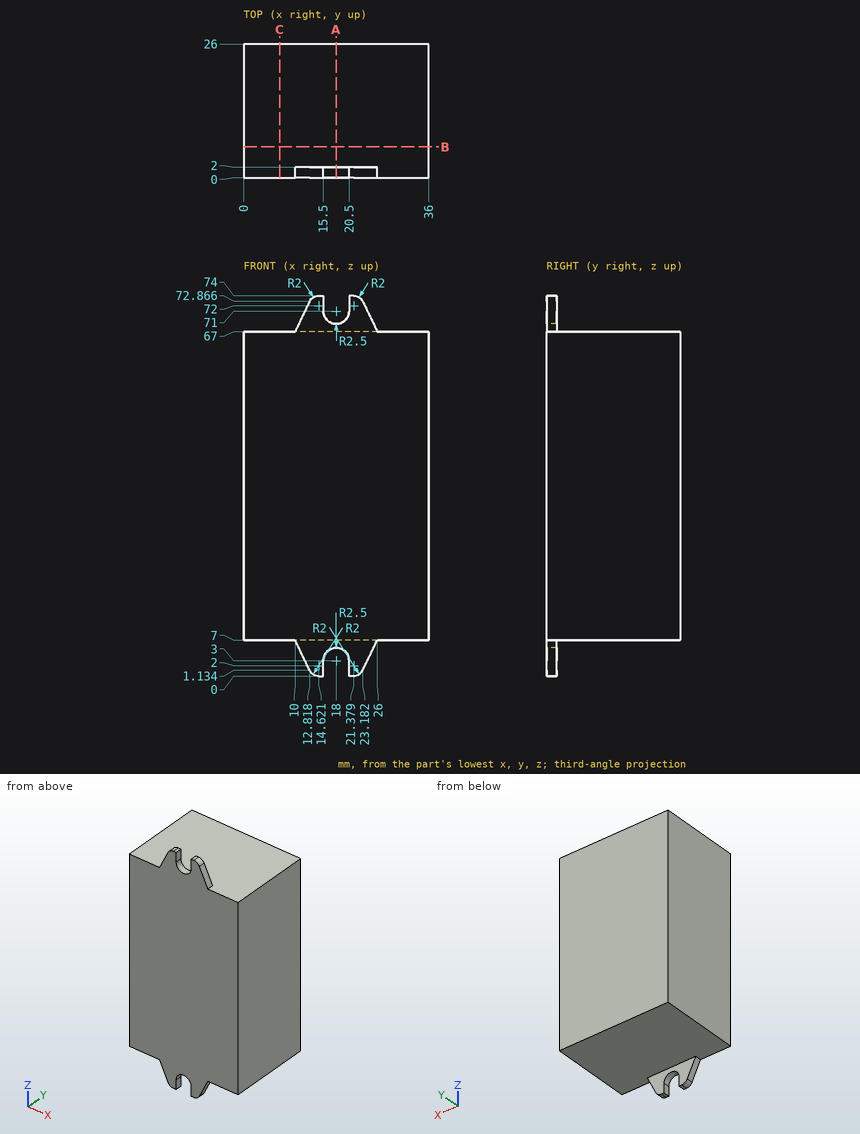
Source: three-view drawing plus pictorial views. Frame: mm from the lowest corner of the part. Round coordinates to 2 decimals unless told otherwise and drop trailing zeros. Order: outer loops, then holes, each group sorted by start corner. A loop starts at its lowest first (then second) coordinate and runs counter-clockwise, first axis right, second up. Notation, with made-up numbers: (47, -0.75) - (85, -0.75) arc R32 cw to (85, 25.25) - close; hole circle Ø11 at (79.25, 9.5). An arc over 180 degrees is marked (long way). Use a Markdown table: item, result.
1. Section C-C on x = 7. Return the cut outline in (y, z).
Evaluation:
| item | result |
|---|---|
| outline | (0, 7) - (26, 7) - (26, 67) - (0, 67) - close |
2. Section B-B on y = 6. Return the cut outline in (x, z), then the cut area to 3 significant figures.
Evaluation:
| item | result |
|---|---|
| outline | (0, 7) - (36, 7) - (36, 67) - (0, 67) - close |
| area | 2,160 mm^2 |
3. Material intervals for probe 1 along Z at (x, y) = (14.5, 7.75), sorted ascending.
Evaluation:
| item | result |
|---|---|
| probe 1 | 7 to 67 |
4. First-contact query: pin 1 (4 mm diameter, centred on x = 17.5, z = 36.5, fed in from -Y); pin 2 (1 mm diameter, centred on y = 1, z = 1.5, fed in from -X); pin 3 (1 mm diameter, centred on x = 20, y = 18, fed in from -Z); pin 4 (0.6 mm diameter, centred on y = 1.5, z = 1.5, fed in from +X). Flat tips, straight axial feed; report the tip coordinate or a pass-through.
Evaluation:
| item | result |
|---|---|
| pin 1 | y = 0 |
| pin 2 | x = 12.4 |
| pin 3 | z = 7 |
| pin 4 | x = 23.5 |
5. Section A-A on x = 18. Return the cut outline in (y, z).
Evaluation:
| item | result |
|---|---|
| outline | (0, 5.5) - (2, 5.5) - (2, 7) - (26, 7) - (26, 67) - (2, 67) - (2, 68.5) - (0, 68.5) - close |
